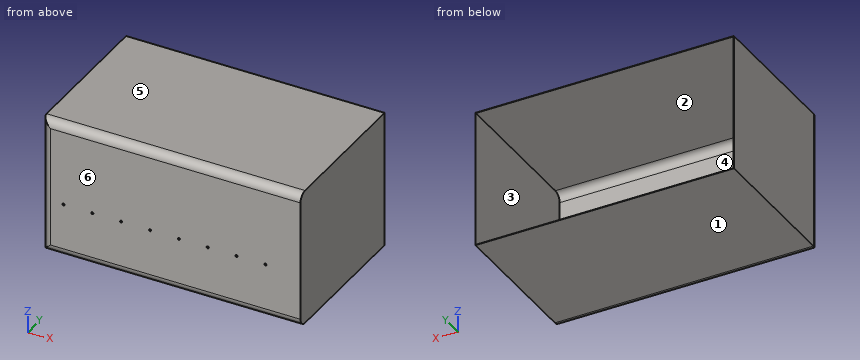
```python
from build123d import *

# Parameters (mm, degrees)
SKETCH1_W           = 780
SKETCH1_H           = 415
BOSS_EXTRUDE1_DEPTH = 460
FILLET1_R           = 25
SHELL1_T            = -1
CUT_EXTRUDE2_REACH  = 998.105
SKETCH2_R           = 3.175


with BuildPart() as part:
    # Sketch1 → Boss-Extrude1 (new body)
    with BuildSketch(Plane(origin=(0, 0, 0), x_dir=(1, 0, 0), z_dir=(0, 1, 0))):
        with Locations((390, -207.5)):
            Rectangle(SKETCH1_W, SKETCH1_H)
    extrude(amount=BOSS_EXTRUDE1_DEPTH)

    # Fillet1
    fillet1_edges = [part.edges().sort_by_distance(p)[0] for p in [
        (390, 0, 0),
        (390, 0, 415),
        (0, 0, 207.5),
    ]]
    fillet(fillet1_edges, radius=FILLET1_R)

    # Shell1
    shell1_openings = [part.faces().sort_by_distance(p)[0] for p in [
        (390, 460, 207.5),
    ]]
    offset(amount=SHELL1_T, openings=shell1_openings)

    # Sketch2 → Cut-Extrude2 (cut, up to next)
    with BuildSketch(Plane.XZ, mode=Mode.PRIVATE) as cut_extrude2_sk1:
        with Locations(Location((65, 164, 0), (0, 0, 270))):
            Circle(SKETCH2_R)
    cut_extrude2_tool1 = extrude(cut_extrude2_sk1.sketch, amount=-CUT_EXTRUDE2_REACH, mode=Mode.PRIVATE) & part.part
    # Sketch2 → Cut-Extrude2 (cut, up to next)
    with BuildSketch(Plane.XZ, mode=Mode.PRIVATE) as cut_extrude2_sk2:
        with Locations(Location((152, 164, 0), (0, 0, 270))):
            Circle(SKETCH2_R)
    cut_extrude2_tool2 = extrude(cut_extrude2_sk2.sketch, amount=-CUT_EXTRUDE2_REACH, mode=Mode.PRIVATE) & part.part
    # Sketch2 → Cut-Extrude2 (cut, up to next)
    with BuildSketch(Plane.XZ, mode=Mode.PRIVATE) as cut_extrude2_sk3:
        with Locations(Location((239, 164, 0), (0, 0, 270))):
            Circle(SKETCH2_R)
    cut_extrude2_tool3 = extrude(cut_extrude2_sk3.sketch, amount=-CUT_EXTRUDE2_REACH, mode=Mode.PRIVATE) & part.part
    # Sketch2 → Cut-Extrude2 (cut, up to next)
    with BuildSketch(Plane.XZ, mode=Mode.PRIVATE) as cut_extrude2_sk4:
        with Locations(Location((326, 164, 0), (0, 0, 270))):
            Circle(SKETCH2_R)
    cut_extrude2_tool4 = extrude(cut_extrude2_sk4.sketch, amount=-CUT_EXTRUDE2_REACH, mode=Mode.PRIVATE) & part.part
    # Sketch2 → Cut-Extrude2 (cut, up to next)
    with BuildSketch(Plane.XZ, mode=Mode.PRIVATE) as cut_extrude2_sk5:
        with Locations(Location((413, 164, 0), (0, 0, 270))):
            Circle(SKETCH2_R)
    cut_extrude2_tool5 = extrude(cut_extrude2_sk5.sketch, amount=-CUT_EXTRUDE2_REACH, mode=Mode.PRIVATE) & part.part
    # Sketch2 → Cut-Extrude2 (cut, up to next)
    with BuildSketch(Plane.XZ, mode=Mode.PRIVATE) as cut_extrude2_sk6:
        with Locations(Location((500, 164, 0), (0, 0, 270))):
            Circle(SKETCH2_R)
    cut_extrude2_tool6 = extrude(cut_extrude2_sk6.sketch, amount=-CUT_EXTRUDE2_REACH, mode=Mode.PRIVATE) & part.part
    # Sketch2 → Cut-Extrude2 (cut, up to next)
    with BuildSketch(Plane.XZ, mode=Mode.PRIVATE) as cut_extrude2_sk7:
        with Locations(Location((587, 164, 0), (0, 0, 270))):
            Circle(SKETCH2_R)
    cut_extrude2_tool7 = extrude(cut_extrude2_sk7.sketch, amount=-CUT_EXTRUDE2_REACH, mode=Mode.PRIVATE) & part.part
    # Sketch2 → Cut-Extrude2 (cut, up to next)
    with BuildSketch(Plane.XZ, mode=Mode.PRIVATE) as cut_extrude2_sk8:
        with Locations(Location((674, 164, 0), (0, 0, 270))):
            Circle(SKETCH2_R)
    cut_extrude2_tool8 = extrude(cut_extrude2_sk8.sketch, amount=-CUT_EXTRUDE2_REACH, mode=Mode.PRIVATE) & part.part
    add(cut_extrude2_tool1.solids().sort_by_distance((65, 0, 164))[0], mode=Mode.SUBTRACT)
    add(cut_extrude2_tool2.solids().sort_by_distance((152, 0, 164))[0], mode=Mode.SUBTRACT)
    add(cut_extrude2_tool3.solids().sort_by_distance((239, 0, 164))[0], mode=Mode.SUBTRACT)
    add(cut_extrude2_tool4.solids().sort_by_distance((326, 0, 164))[0], mode=Mode.SUBTRACT)
    add(cut_extrude2_tool5.solids().sort_by_distance((413, 0, 164))[0], mode=Mode.SUBTRACT)
    add(cut_extrude2_tool6.solids().sort_by_distance((500, 0, 164))[0], mode=Mode.SUBTRACT)
    add(cut_extrude2_tool7.solids().sort_by_distance((587, 0, 164))[0], mode=Mode.SUBTRACT)
    add(cut_extrude2_tool8.solids().sort_by_distance((674, 0, 164))[0], mode=Mode.SUBTRACT)


solid = part.part
```
Check sheet for the modelled part. Datum: model origin and axes. Units: mm. Face numbers are marked on the shaded views. A direction names the side the tool comes from. Round coordinates to 2 decimals unless told otherwise and drop trailing zeros. Write each loop counter-clockwise with the first axis right and the second up, starting at its lowest first coordinate (ties: lowest second). Pieces come first, ordered by that corner, then holes. Notation, with made-up numbers: (-3.5, 2.5) -> (8.5, 2.5) arc R18 cw to (8.5, 6.5) -> close; hole circle Ø8 at (58, 37.25). An arc over 180 degrees is marked (long way). One line per question, with ' | ' between items. Start each with the question number.
1. Release check for a two-part mould opening along Z. For the marked faces 3, 4, 5 and 6 record: +Z half, -Z half, draft (parallel to the pull), parting line (faces both ways), or undercut.
2. Scan lines: line 1 along Z through (x, y) = (260, 341); line 2 along X through (y, z) = (186.5, 37); line 3 along Y through (x, z) = (388, 353.5). Record each from-to range of solid material in increasing order. Write a range as from..to.
3. Sectioned sample at B-B, the plane z = 346.5. Record the cut outline in (x, y), then the cut area to 3 significant figures.
4. Sectioned sample at C-C, the plane x = 121.5. Record the cut outline in (y, z).
5. Depth check by flat-ended pin: pin 1 (8.5 mm diameter, centred on x = 152, z = 164, fed in from +Y); pin 2 (4 mm diameter, centred on x = 587, z = 164, fed in from -Y). Enter the tip coordinate at first touch or a pass-through.
6. Sectioned sample at A-A, the plane y = 120. Record the cut outline in (x, z).
7. Set-up check for the marked faces 1 and 2: record each of +Z, -Z, +X, -X, +Y, -Y from which the full face is reachable in a straight line by a thin tool's end or side.
Taken from the geometry:
1) face 3: undercut | face 4: undercut | face 5: +Z half | face 6: draft
2) line 1: z = 0..1, 414..415 | line 2: x = 0..1, 779..780 | line 3: y = 0..1
3) outline: (0, 25) arc R25 ccw to (25, 0) -> (780, 0) -> (780, 460) -> (779, 460) -> (779, 1) -> (25, 1) arc R24 cw to (1, 25) -> (1, 460) -> (0, 460) -> close | area: 1,690 mm^2
4) outline: (0, 25) arc R25 ccw to (25, 0) -> (460, 0) -> (460, 1) -> (25, 1) arc R24 cw to (1, 25) -> (1, 390) arc R24 cw to (25, 414) -> (460, 414) -> (460, 415) -> (25, 415) arc R25 ccw to (0, 390) -> close
5) pin 1: stops at y = 1 | pin 2: passes through
6) outline: (0, 0) -> (780, 0) -> (780, 415) -> (0, 415) -> close; hole (1, 1) -> (779, 1) -> (779, 414) -> (1, 414) -> close
7) face 1: -Z, +X, -X, +Y, -Y | face 2: +Y
